CAD build for the part. Positions are in the model's coordinates, mm. Face numbers are marked on the shaded views. Give positions to 0.01 mm unless a question says otherwise; leave off trailing zeros. Write each loop counter-clockwise with the first axis right and the second up, starting at its lowest first coordinate (ties: lowest second). Pieces come first, ordered by that corner, then holes. Notation, with made-up numbers: (-18, 88) -> (10, 88) arc R30 ccw to (10, 122) -> close; hole circle Ø4 at (-25, 25.25). An arc over 180 degrees is marked (long way). Answer in a Markdown table with one row per item. Add a question column.
```python
from build123d import *

# Parameters (mm, degrees)
F0_R        = 17.6278331086
F1_DEPTH    = 6.858
F2_T1_DEPTH = 21.5226968374


# Not quite as in the source:
# - a fillet or chamfer that OpenCascade refuses, or shapes differently, is made with other operations: its cross-section is extruded or revolved along the edge and cut away or added


with BuildPart() as f1:
    # F0 (on Front) → F1 (new body)
    with BuildSketch(Plane.XZ):
        Polygon((25.0675420445, 0.0543576147), (12.486695947, 21.7363070283), (-12.5808460975, 21.6819494136), (-25.0675420445, -0.0543576147), (-12.486695947, -21.7363070283), (12.5808460975, -21.6819494136), align=None)
        Circle(F0_R, mode=Mode.SUBTRACT)
    extrude(amount=F1_DEPTH)

    # F2: fillet of radius 5.08 on 7 edges, made by hand

    # F2_s2 → F2_t1 (cut)
    with BuildSketch(Plane.XZ.offset(-7.3323484187)):
        with BuildLine():
            ThreePointArc((-23.6065836488, 2.4888163666), (-24.2816651572, -0.052653483), (-23.5955679683, -2.5911716899))
            Line((-23.5955679683, -2.5911716899), (-25.0675420445, -0.0543576147))
            Line((-25.0675420445, -0.0543576147), (-23.6065836488, 2.4888163666))
        make_face()
        with BuildLine():
            ThreePointArc((-13.9586700232, -19.1994929531), (-12.0952333247, -21.0548656138), (-9.5537634751, -21.7299471223))
            Line((-9.5537634751, -21.7299471223), (-12.486695947, -21.7363070283))
            Line((-12.486695947, -21.7363070283), (-13.9586700232, -19.1994929531))
        make_face()
        with BuildLine():
            ThreePointArc((14.0418044932, -19.1387754323), (12.1864318325, -21.0022121308), (9.6479136256, -21.6883093197))
            Line((9.6479136256, -21.6883093197), (12.5808460975, -21.6819494136))
            Line((12.5808460975, -21.6819494136), (14.0418044932, -19.1387754323))
        make_face()
        with BuildLine():
            ThreePointArc((23.6065836488, -2.4888163666), (24.2816651572, 0.052653483), (23.5955679683, 2.5911716899))
            Line((23.5955679683, 2.5911716899), (25.0675420445, 0.0543576147))
            Line((25.0675420445, 0.0543576147), (23.6065836488, -2.4888163666))
        make_face()
        with BuildLine():
            ThreePointArc((13.9586700232, 19.1994929531), (12.0952333247, 21.0548656138), (9.5537634751, 21.7299471223))
            Line((9.5537634751, 21.7299471223), (12.486695947, 21.7363070283))
            Line((12.486695947, 21.7363070283), (13.9586700232, 19.1994929531))
        make_face()
        with BuildLine():
            ThreePointArc((-9.6479136256, 21.6883093197), (-12.1864318325, 21.0022121308), (-14.0418044932, 19.1387754323))
            Line((-14.0418044932, 19.1387754323), (-12.5808460975, 21.6819494136))
            Line((-12.5808460975, 21.6819494136), (-9.6479136256, 21.6883093197))
        make_face()
    extrude(amount=F2_T1_DEPTH, mode=Mode.SUBTRACT)

    # F2_s3 → F2_t4 (revolve, cut)
    with BuildSketch(Plane.XY):
        with BuildLine():
            ThreePointArc((17.6278331086, -1.778), (19.1157306602, -5.3701024484), (22.7078331086, -6.858))
            Line((22.7078331086, -6.858), (17.6278331086, -6.858))
            Line((17.6278331086, -6.858), (17.6278331086, -1.778))
        make_face()
    revolve(axis=Axis((0, -6.858, 0), (0, -1, 0)), mode=Mode.SUBTRACT)


solid = f1.part
```
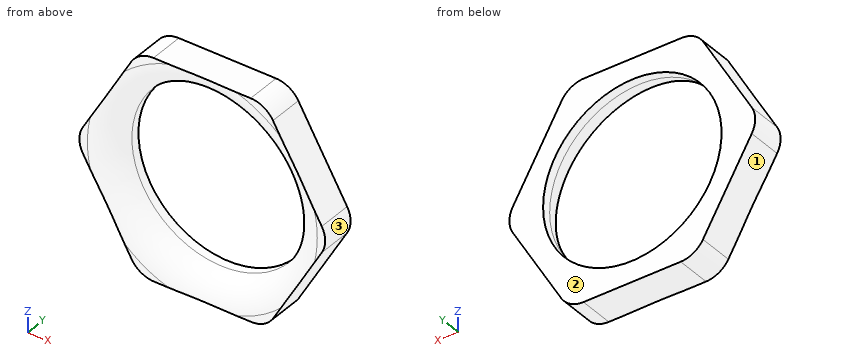
Item 1: Slice it at D-D, the plane y = -3.5. List the corners of the cut face in (x, z).
Item 2: Drop flat-ended pins along their axis: pin 1 Ø6 at (x, z) = (-18, 2.5) entering from -Y; pin 2 Ø4 at (x, z) = (-14, -2.5) entering from +Y; pin 3 Ø3 at (y, z) = (-5, 9) entering from +X; pin 4 Ø1 at (x, y) = (4, -3.5) entering from -Z. Give the stop position or say it passes through.
Item 3: Slice it at A-A, the plane y = -0.75. List the corners of the cut face in (x, z).
Item 4: Slice it at C-C, the plane x = 0. List the corners of the cut face in (y, z).
Item 5: Mould opens along X. For the marked faces 1, 2 and 3 say: released by +X, released by -X, zero draft, split by the parting line, or undercut.
Item 6: Probe L1, parallel to Z at x = -19.5, y = -1.25; L2, parallel to Z at x = 0, y = -4; L3, parallel to Z at x = -16.5, y = -3.5. List the from-to ranges inside material, lowest first. Write a range as from..to.
Item 7: Slice it at B-B, the plane z = 0. List the corners of the cut face in (x, y).
Answer key:
| question | item | result |
|---|---|---|
| 1 | outline | (-23.61, 2.49) arc R5.08 ccw to (-23.6, -2.59) -> (-13.96, -19.2) arc R5.08 ccw to (-9.55, -21.73) -> (9.65, -21.69) arc R5.08 ccw to (14.04, -19.14) -> (23.61, -2.49) arc R5.08 ccw to (23.6, 2.59) -> (13.96, 19.2) arc R5.08 ccw to (9.55, 21.73) -> (-9.65, 21.69) arc R5.08 ccw to (-14.04, 19.14) -> close; hole circle Ø35.86 at (0, 0) |
| 2 | pin 1 | stops at y = -6.62 |
| 2 | pin 2 | passes through |
| 2 | pin 3 | stops at x = 20.75 |
| 2 | pin 4 | stops at z = -21.7 |
| 3 | outline | (-23.61, 2.49) arc R5.08 ccw to (-23.6, -2.59) -> (-13.96, -19.2) arc R5.08 ccw to (-9.55, -21.73) -> (9.65, -21.69) arc R5.08 ccw to (14.04, -19.14) -> (23.61, -2.49) arc R5.08 ccw to (23.6, 2.59) -> (13.96, 19.2) arc R5.08 ccw to (9.55, 21.73) -> (-9.65, 21.69) arc R5.08 ccw to (-14.04, 19.14) -> close; hole circle Ø35.26 at (0, 0) |
| 4 | outline | (-6.76, -21.71) -> (0, -21.71) -> (0, -17.63) -> (-1.78, -17.63) arc R5.08 ccw to start; (-6.76, 21.71) arc R5.08 ccw to (-1.78, 17.63) -> (0, 17.63) -> (0, 21.71) -> close |
| 5 | face 1 | released by -X |
| 5 | face 2 | zero draft |
| 5 | face 3 | released by +X |
| 6 | L1 | z = -9.65..9.64 |
| 6 | L2 | z = -21.71..-18.14, 18.14..21.71 |
| 6 | L3 | z = -14.82..-7.01, 7.01..14.86 |
| 7 | outline | (-24.28, -6.86) -> (-22.71, -6.86) arc R5.08 ccw to (-17.63, -1.78) -> (-17.63, 0) -> (-24.28, 0) -> close; (17.63, -1.78) arc R5.08 ccw to (22.71, -6.86) -> (24.28, -6.86) -> (24.28, 0) -> (17.63, 0) -> close |
